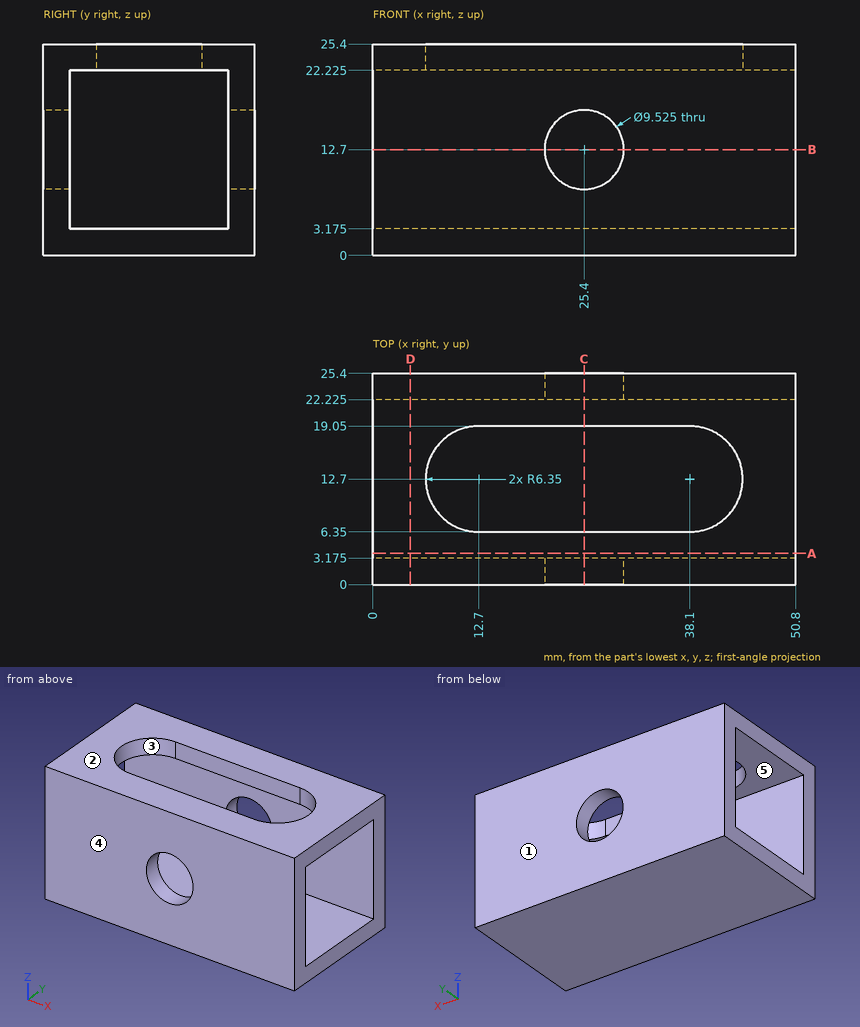
For this review, use the dimensioned drawing (mm, ordinates from the lowest corner) and the shaded views. A direction names the side the tool comes from. Give positions to 0.01 mm unless a question says otherwise; leave off trailing zeros. Write each loop counter-clockwise with the first axis right and the second up, starting at its lowest first coordinate (ties: lowest second). Pieces come first, ordered by that corner, then holes. Notation, with made-up numbers: M -33.5,-24.75 L 0.5,-24.75 A18 ccw 0.5,3.25 Z; hole C 89.5,49 d9. An arc over 180 degrees is marked long. Write item = value, one per line. Start each with the question number.
Q1. We need section A-A (y = 3.75). State the section outline as (x, z) points (3 decimals), plus the area to 3 significant figures.
Q2. Mouldability with a two-part tool opening along Y and no side actions: class the marked faces 1, 2 and 3 as released by +Y, released by -Y, zero draft, split by the parting line, or undercut.
Q3. We need section C-C (x = 25.4). Give the number of separate pieces and of enclosed holes in the cut face, plus the area to 3 significant figures.
Q4. Machinability: for the marked faces 4 and 5, which of the approach directions +Z, -Z, +X, -X, +Y, -Y give a long, thin tool a straight path to every point of the face, cutting with its end or side? Answer none if there is none.
Q5. Clearance check with flat-ended pins moving along their axes: pin 1 (6 mm diameter, centred on x = 36.5, y = 15.5, fed in from +Z) (3 decimals); pin 2 (1.5 mm diameter, centred on y = 20, z = 10, fed in from -X). State where each tip first meets the part, or that it passes through.
Q6. We need section B-B (z = 12.7). State the section outline as (x, y) points (1 decimal), plus the area to 3 significant figures.
Q7. We need section D-D (x = 4.5). State the section outline as (y, z) points (3 decimals).
Q8. For line 1 (Z direction, x = 25.4, y = 2.4); line 2 (Y direction, x = 42.5, z = 12) (3 decimals), list the stretches that pass through material, from the lowest coordinate up.
Result set:
q1.outline = M 0,0 L 50.8,0 L 50.8,3.175 L 0,3.175 Z; M 0,22.225 L 50.8,22.225 L 50.8,25.4 L 0,25.4 Z
q1.area = 323 mm2
q2.face_1 = released by +Y
q2.face_2 = zero draft
q2.face_3 = undercut
q3.separate_pieces = 3
q3.enclosed_holes = 0
q3.area = 181 mm2
q4.face_4 = +Z, -Z, +X, -X, -Y
q4.face_5 = +X, -X
q5.pin_1 = 3.175
q5.pin_2 = through
q6.outline = M 0,0 L 20.6,0 L 20.6,3.2 L 0,3.2 Z; M 0,22.2 L 20.6,22.2 L 20.6,25.4 L 0,25.4 Z; M 30.2,0 L 50.8,0 L 50.8,3.2 L 30.2,3.2 Z; M 30.2,22.2 L 50.8,22.2 L 50.8,25.4 L 30.2,25.4 Z
q6.area = 262 mm2
q7.outline = M 0,0 L 25.4,0 L 25.4,25.4 L 0,25.4 Z; hole M 3.175,3.175 L 22.225,3.175 L 22.225,22.225 L 3.175,22.225 Z
q8.line_1 = 0 to 7.94, 17.46 to 25.4
q8.line_2 = 0 to 3.175, 22.225 to 25.4
